Autodesk Inventor part; units mm, degrees
ref_plane "Plan YZ" through (0, 0, 0) normal (1, 0, 0) x (0, 1, 0)
ref_plane "Plan XZ" through (0, 0, 0) normal (0, 1, 0) x (-1, 0, 0)
ref_plane "Plan XY" through (0, 0, 0) normal (0, 0, 1) x (1, 0, 0)
sketch "Esquisse12" plane through (0, 0, 0) normal (0, 0, 1) x (1, 0, 0)
  line L0 (-88, -26) -> (-88, 26)
  line L1 (-88, 26) -> (-83, 26)
  line L2 (-83, 26) -> (-83, 29)
  line L3 (-83, 29) -> (-68, 29)
  line L4 (-68, 29) -> (-68, 26)
  line L5 (7.5, 26) -> (7.5, 29)
  line L6 (7.5, 29) -> (-7.5, 29)
  line L7 (-7.5, 29) -> (-7.5, 26)
  line L8 (68, 26) -> (68, 29)
  line L9 (68, 29) -> (83, 29)
  line L10 (83, 29) -> (83, 26)
  line L11 (83, 26) -> (88, 26)
  line L12 (88, 26) -> (88, -26)
  line L13 (88, -26) -> (83, -26)
  line L14 (83, -26) -> (83, -29)
  line L15 (83, -29) -> (68, -29)
  line L16 (68, -29) -> (68, -26)
  line L17 (-7.5, -26) -> (-7.5, -29)
  line L18 (7.5, -29) -> (7.5, -26)
  line L19 (-68, -26) -> (-68, -29)
  line L20 (-83, -29) -> (-83, -26)
  line L21 (-88, -26) -> (-83, -26)
  line L22 (-83, -29) -> (-68, -29)
  line L23 (7.5, -29) -> (-7.5, -29)
  line L24 (-68, 26) -> (-7.5, 26)
  line L25 (7.5, 26) -> (68, 26)
  line L26 (7.5, -26) -> (68, -26)
  line L27 (-7.5, -26) -> (-68, -26)
  line L28 (-123.2, 0) -> (123.2, 0) construction
  line L29 (0, -40.6) -> (0, 40.6) construction
  point P0 (0, 0)
  dimension "d86" = 52
  dimension "d87" = 3
  dimension "d88" = 5
  dimension "d90" = 15
  dimension "d112" = 176
extrude "Extrusion5" add sketch "Esquisse12" along normal blind 3
sketch "Esquisse13" plane through (0, 0, 3) normal (0, 0, 1) x (1, 0, 0)
  point P0 (0, 0)
  point P1 (-83, 26)
  point P2 (-68, 26)
  point P3 (-83, -26)
  point P4 (-68, -26)
  point P5 (-7.5, -26)
  point P6 (7.5, -26)
  point P7 (68, -26)
  point P8 (83, -26)
  point P9 (83, 26)
  point P10 (68, 26)
  point P11 (-7.5, 26)
  point P12 (7.5, 26)
hole "Perçage6" at (-83, 26, 3) at (-68, 26, 3) at (-83, -26, 3) at (-68, -26, 3) at (-7.5, -26, 3) at (7.5, -26, 3) at (68, -26, 3) at (83, -26, 3) at (83, 26, 3) at (68, 26, 3) at (-7.5, 26, 3) at (7.5, 26, 3) direction (0, 0, -1) diameter 1 end through all
chamfer "Chanfrein3" distance 1 angle 45 12 edges at (-83, 29, 1.5) (-68, 29, 1.5) (-7.5, 29, 1.5) (7.5, 29, 1.5) (68, 29, 1.5) (83, 29, 1.5) (-83, -29, 1.5) (-68, -29, 1.5) (-7.5, -29, 1.5) (7.5, -29, 1.5) (68, -29, 1.5) (83, -29, 1.5)
sketch "Esquisse14" plane through (0, 0, 3) normal (0, 0, 1) x (1, 0, 0)
  circle A0 centre (16.2, 13.8) radius 5
  line L0 (-88, -26) -> (-88, 26)
  line L1 (67.5, -26) -> (8, -26)
  line L2 (88, 26) -> (88, -26)
  point P0 (0, 0)
  dimension "d108" = 39.8
  dimension "d109" = 10
  dimension "d113" = 71.8
extrude "Extrusion6" cut sketch "Esquisse14" against normal through all
properties part number "P1704_103" material "Plastique PMMA"
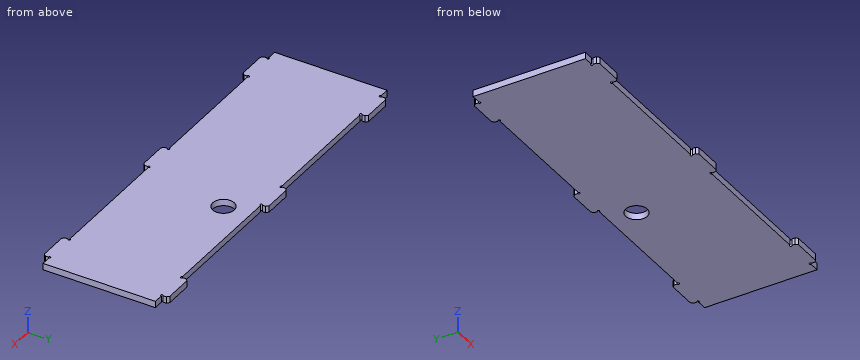
Design review of the part built by this model. Coordinates are the model's own, in mm. Round coordinates to 2 decimals unless told otherwise and drop trailing zeros. Write each loop counter-clockwise with the first axis right and the second up, starting at its lowest first coordinate (ties: lowest second). Pieces come first, ordered by that corner, then holes. Notation, with made-up numbers: (-23, -34) -> (10, -34) arc R21 ccw to (10, -27) -> close; hole circle Ø2 at (31, 61). An arc over 180 degrees is marked (long way). Write item = value, one per line. Start each with the question number.
1) Take a section at A-A, the plane y = 11. State the section outline as (x, z) points, plus the area to 3 significant figures.
2) Clearance check with flat-ended pins moving along their axes: pin 1 (0.9 mm diameter, centred on x = 85, z = 1.5, fed in from +Y); pin 2 (0.8 mm diameter, centred on y = 27, z = 2, fed in from -X); pin 3 (0.9 mm diameter, centred on x = -24.5, z = 1.5, fed in from -Y). State where each tip first meets the part, or that it passes through.
3) Wall thickness on probe 1 along Y at (x, z) = (62.5, 1.65); probe 2 along Y at (x, z) = (13.5, 2.4); probe 3 along Y at (x, z) = (12.5, 1.5): over which ranges is each line inside the solid? List them lowest first. Write a range as from..to.
4) Take a section at B-B, the plane x = -47.5. State the section outline as (y, z) points.
Results list:
q1.outline = (-88, 0) -> (12.06, 0) -> (12.06, 3) -> (-88, 3) -> close; (20.34, 0) -> (88, 0) -> (88, 3) -> (20.34, 3) -> close
q1.area = 503 mm²
q2.pin_1 = 26
q2.pin_2 = -83
q2.pin_3 = -26
q3.probe_1 = -26..26
q3.probe_2 = -26..9.59, 18.01..26
q3.probe_3 = -26..10.44, 17.16..26
q4.outline = (-26, 0) -> (26, 0) -> (26, 3) -> (-26, 3) -> close
